Drawing for the job (mm, zero at the part's lowest x, y, z). Round coordinates to 2 decimals unless told otherwise and drop trailing zeros. Order: outer loops, then holes, each group sorted by start corner. A loop starts at its lowest first (then second) coordinate and runs counter-clockwise, first axis right, second up. Notation, with made-up numbers: M 25.25,60.25 L 52.25,60.25 A10 ccw 52.25,76.25 Z; hole C 0,-19 d3. An arc over 180 degrees is marked long. One line per item, written item: value. Start each with the question number.
Item 1: Band-saw the part on D-D, the plane z = 37. Write the cut outline in (x, y).
Item 2: Pin check, flat tips, straight feed: pin 1 (1.5 mm diameter, centred on y = 52, z = 33.5, fed in from -X); pin 2 (1 mm diameter, centred on x = 27.5, y = 71.5, fed in from +Z); pin 3 (1.5 mm diameter, centred on x = 28, y = 40.5, fed in from -Z). Stop position of each tip, or through.
Item 3: Probe L1, parallel to Y at x = 42, z = 5.5; L2, parallel to X at y = 71.5, z = 42.5; L3, parallel to X at y = 53, z = 21.5. List the from-to ranges inside material, lowest first.
Item 4: Two-plate mould, pull along X, no slides. Class the marked faces 1 and 2: +X half, -X half, draft (parallel to the pull), parting line (faces both ways), or undercut.
Item 5: Band-saw the part on C-C, the plane z = 10.5. Write the cut outline in (x, y), then the cut area to 3 significant figures.
Item 6: Band-saw the part on A-A, the plane x = 42. Write the cut outline in (y, z).
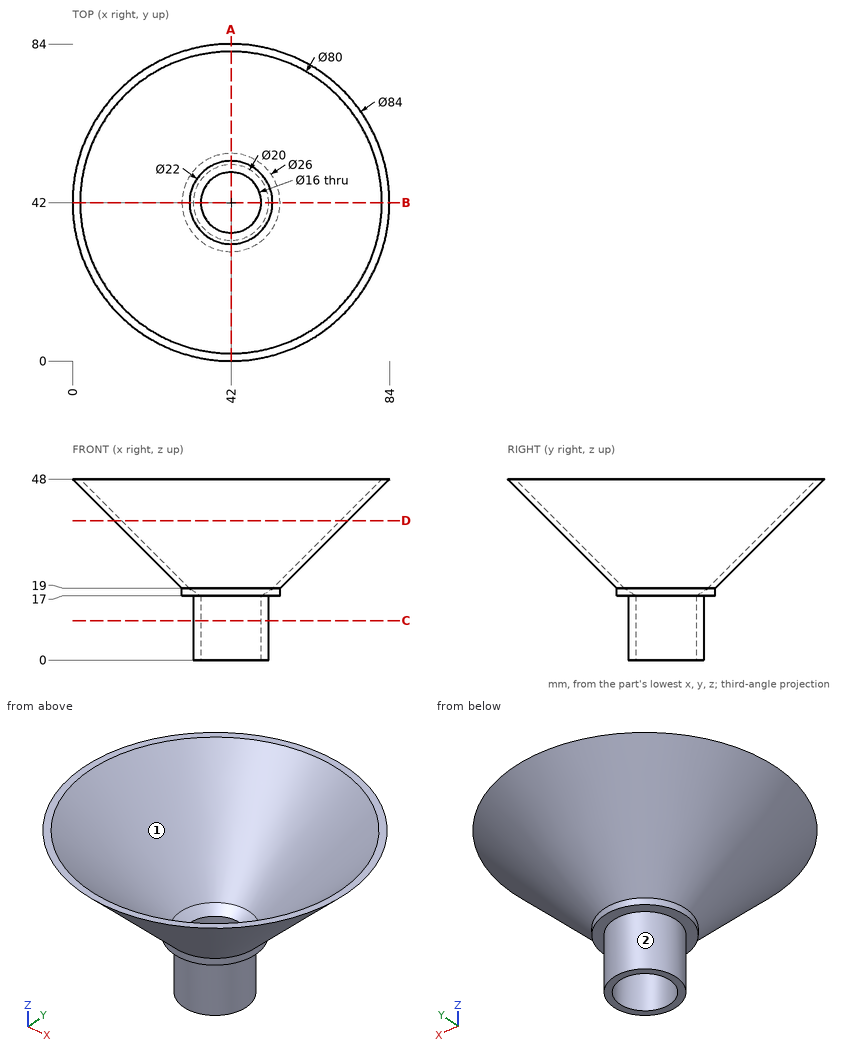
Output:
1. outline: C 42,42 d62; hole C 42,42 d58
2. pin 1: stops at x = 15.53
2. pin 2: stops at z = 41.37
2. pin 3: stops at z = 19.33
3. L1: y = 32 to 34, 50 to 52
3. L2: x = 20.51 to 24.11, 59.89 to 63.49
3. L3: x = 31.08 to 34.17, 49.83 to 52.92
4. face 1: undercut
4. face 2: parting line
5. outline: C 42,42 d20; hole C 42,42 d16
5. area: 113 mm²
6. outline: M 0,48 L 29,19 L 29,17 L 32,17 L 32,0 L 34,0 L 34,17 L 31,19 L 2,48 Z; M 50,0 L 52,0 L 52,17 L 55,17 L 55,19 L 84,48 L 82,48 L 53,19 L 50,17 Z
